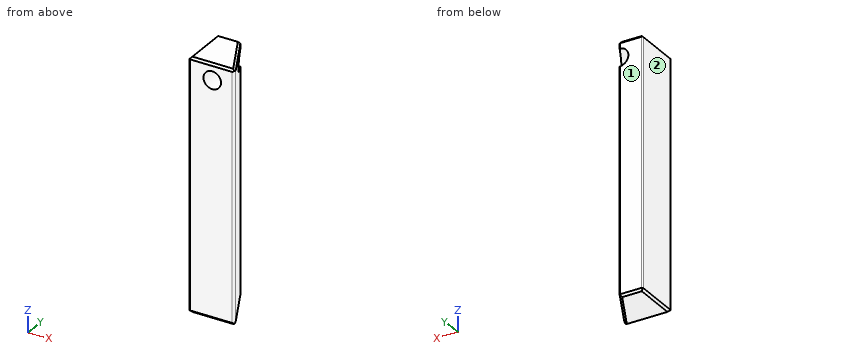
from build123d import *

# Parameters (mm, degrees)
BASE_DEPTH        = 60.25
FACE_CHAMFER_SIZE = 0.5
SMALLER_FILLETS_R = 0.25
LARGER_FILLET_R   = 0.5
SKETCH2_R         = 2.11
HOLE_DEPTH        = 63.216278519


with BuildPart() as part:
    # Sketch1 → Base (new body)
    with BuildSketch(Plane.XY):
        Polygon((0, 11.15), (0, 0), (11.1, 0), (5.55, 11.15), align=None)
    extrude(amount=BASE_DEPTH)

    # Face Chamfer
    face_chamfer_edges = [part.edges().sort_by_distance(p)[0] for p in [
        (5.55, 0, 60.25),
        (8.325, 5.575, 60.25),
        (2.775, 11.15, 60.25),
        (8.325, 5.575, 0),
        (5.55, 0, 0),
        (0, 5.575, 0),
        (2.775, 11.15, 0),
        (0, 5.575, 60.25),
    ]]
    chamfer(face_chamfer_edges, length=FACE_CHAMFER_SIZE)

    # Smaller Fillets
    smaller_fillets_edges = [part.edges().sort_by_distance(p)[0] for p in [
        (0, 0, 30.125),
        (0, 11.15, 30.125),
        (5.55, 11.15, 30.125),
    ]]
    fillet(smaller_fillets_edges, radius=SMALLER_FILLETS_R)

    # Larger Fillet
    larger_fillet_edges = [part.edges().sort_by_distance(p)[0] for p in [
        (11.1, 0, 30.125),
    ]]
    fillet(larger_fillet_edges, radius=LARGER_FILLET_R)

    # Sketch2 → Hole (cut, through all)
    with BuildSketch(Plane(origin=(0, 11.15, 0), x_dir=(1, 0, 0), z_dir=(0, 1, 0))):
        with Locations(Location((5.55, -56.39, 0), (0, 0, 180))):
            Circle(SKETCH2_R)
    extrude(amount=-HOLE_DEPTH, mode=Mode.SUBTRACT)


solid = part.part
Build history of the part. All positions in model axes, mm. Face numbers are marked on the shaded views. Coordinates: 2 decimals unless noted, no trailing zeros. Order: outer loops, then holes, each group sorted by start corner. A loop starts at its lowest first (then second) coordinate and runs counter-clockwise, first axis right, second up. Notation, with made-up numbers: (-14.5, 24) - (23.5, 24) arc R15 ccw to (23.5, 43) - close; hole circle Ø5 at (22, 39). An arc over 180 degrees is marked (long way). Put each result on its own line as item: value.
1. Drop flat-ended pins along their axis: P1, Ø3.5, axis at x = 5.55, z = 56.39, coming from the -Y side; P2, Ø5, axis at x = 9.5, z = 53.5, coming from the +Y side; P3, Ø6, axis at y = 4.5, z = 19, coming from the +X side. Give the stop position or say it passes through.
Answer sheet:
P1: passes through
P2: stops at y = 8.24
P3: stops at x = 10.35
2. Saw through at A-A (x = 6.5). Write the cut outline in (y, z).
Answer sheet:
outline: (0, 0.5) - (0.5, 0) - (8.12, 0) - (9.24, 0.5) - (9.24, 54.51) - (0, 54.51) - close; (0, 58.27) - (9.24, 58.27) - (9.24, 59.75) - (8.12, 60.25) - (0.5, 60.25) - (0, 59.75) - close
3. Saw through at B-B (z = 56.39). Write the cut outline in (x, y), and give its area (3 significant figures).
Answer sheet:
outline: (0, 0.25) arc R0.25 ccw to (0.25, 0) - (3.44, 0) - (3.44, 11.15) - (0.25, 11.15) arc R0.25 ccw to (0, 10.9) - close; (7.66, 0) - (10.29, 0) arc R0.5 ccw to (10.74, 0.72) - (7.66, 6.91) - close
area: 50.1 mm^2
4. Saw through at D-D (z = 37). Write the cut outline in (x, y).
Answer sheet:
outline: (0, 0.25) arc R0.25 ccw to (0.25, 0) - (10.29, 0) arc R0.5 ccw to (10.74, 0.72) - (5.62, 11.01) arc R0.25 ccw to (5.4, 11.15) - (0.25, 11.15) arc R0.25 ccw to (0, 10.9) - close
5. Saw through at C-C (y = 5). Write the cut outline in (x, z), and give its area (3 significant figures).
Answer sheet:
outline: (0, 0.5) - (0.5, 0) - (8.05, 0) - (8.61, 0.5) - (8.61, 59.75) - (8.05, 60.25) - (0.5, 60.25) - (0, 59.75) - close; hole circle Ø4.22 at (5.55, 56.39)
area: 504 mm^2
6. Probe line 1 along Z through (x, y) = (5.55, 8.75); line 2 along X through (y, z) = (5.5, 56.39); line 3 along X through (y, z) = (5, 56.39). List the from-to ranges inside material, lowest first. Write a range as [from, to].
Answer sheet:
line 1: z = [0, 54.28], [58.5, 60.25]
line 2: x = [0, 3.44], [7.66, 8.36]
line 3: x = [0, 3.44], [7.66, 8.61]
7. Pull direction X, two halves, no side cores. Call the marked faces 1 and 2: pulls with the +X half, pulls with the -X half, needs draft (parallel to the pull), parting line crosses it, or undercut.
Answer sheet:
face 1: needs draft
face 2: pulls with the -X half
